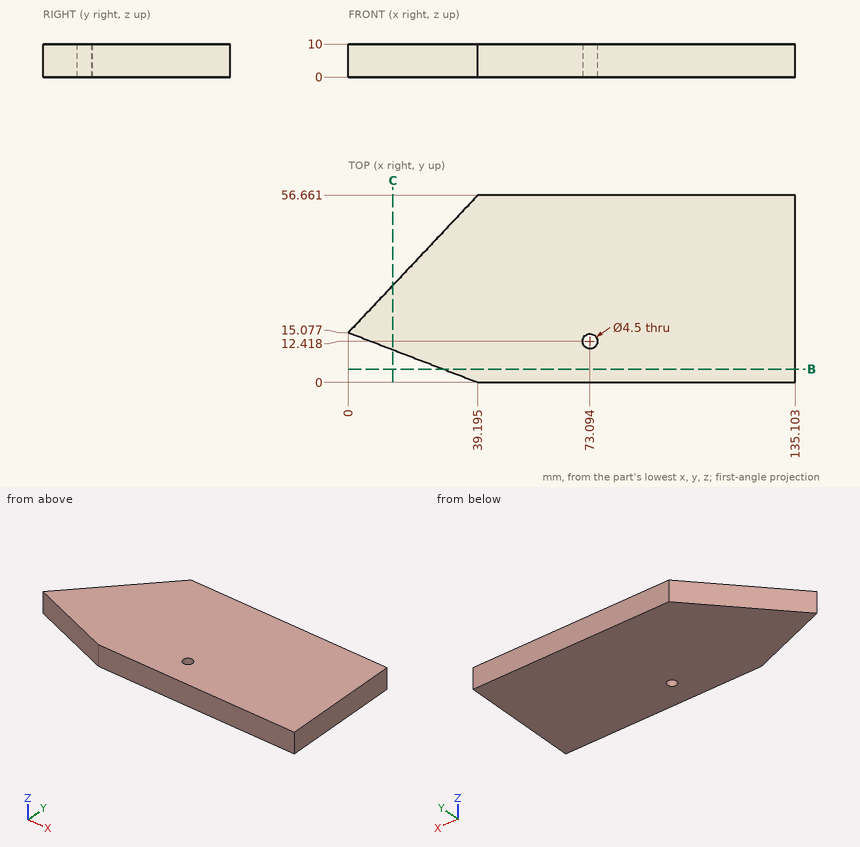
For this review, use the dimensioned drawing (mm, ordinates from the lowest corner) and the shaded views. Give positions to 0.01 mm unless a question says otherwise; leave off trailing zeros. Order: outer loops, then holes, each group sorted by start corner. A loop starts at its lowest first (then second) coordinate and runs counter-clockwise, first axis right, second up. Notation, with made-up numbers: (-19.75, 29.5) - (11.25, 29.5) arc R19 cw to (11.25, 60.5) - close; hole circle Ø9 at (87.5, -10.75). An arc over 180 degrees is marked (long way). Use CSV: the item, a comma, the result in double quotes. Start each with the question number.
Q1. To check wall thickness, follow line 1 along X through (y, z) = (44, 7.5) (1 decimal); line 2 along X through (y, z) = (43.5, 8.5) (1 decimal); line 3 along Y through (x, z) = (28, 9.75) (1 decimal). State the ranges of each line that lie inside material, in increasing order. Write a range as [from, to].
Q2. We need section B-B, the plane y = 4. Write out the cut boundary in (x, z), and give its area (3 significant figures).
Q3. We need section C-C, the plane x = 13.5. Write out the cut boundary in (y, z).
Outcome:
1,line 1,"x = [27.3, 135.1]"
1,line 2,"x = [26.8, 135.1]"
1,line 3,"y = [4.3, 44.8]"
2,outline,"(28.8, 0) - (135.1, 0) - (135.1, 10) - (28.8, 10) - close"
2,area,"1,060 mm^2"
3,outline,"(9.88, 0) - (29.4, 0) - (29.4, 10) - (9.88, 10) - close"
